Design review of the part built by this model. Coordinates are the model's own, in mm. Face numbers are marked on the shaded views. A direction names the side the tool comes from. Coordinates: 2 decimals unless noted, no trailing zeros. Order: outer loops, then holes, each group sorted by start corner. A loop starts at its lowest first (then second) coordinate and runs counter-clockwise, first axis right, second up. Notation, with made-up numbers: (-33, 39.25) - (19, 39.25) arc R8 ccw to (19, 48.25) - close; hole circle Ø4 at (46, 44). An arc over 180 degrees is marked (long way). Write each question's results on one line, items separated by ' | '. Start each with the question number.
```python
from build123d import *

# Parameters (mm, degrees)
SKETCH3_W           = 42.3
SKETCH3_H           = 42.3
BOSS_EXTRUDE1_DEPTH = 20.95
SKETCH4_R           = 4.05
CUT_EXTRUDE1_DEPTH  = 5
SKETCH5_R           = 2.5
CUT_EXTRUDE2_DEPTH  = 8.5
SKETCH6_R           = 3.05
BOSS_EXTRUDE2_DEPTH = 5
SKETCH7_R           = 2.05
CUT_EXTRUDE3_DEPTH  = 20
CHAMFER1_SIZE       = 4
CHAMFER3_SIZE       = 1
CUT_EXTRUDE4_DEPTH  = 1


with BuildPart() as part:
    # Sketch3 → Boss-Extrude1 (new body)
    with BuildSketch(Plane.XY):
        Rectangle(SKETCH3_W, SKETCH3_H)
    extrude(amount=BOSS_EXTRUDE1_DEPTH)

    # Sketch4 → Cut-Extrude1 (cut)
    with BuildSketch(Plane.XZ.offset(21.15)):
        with Locations(Location((0, 12.45, 0), (0, 0, 270))):
            Circle(SKETCH4_R)
    extrude(amount=-CUT_EXTRUDE1_DEPTH, mode=Mode.SUBTRACT)

    # Sketch5 → Cut-Extrude2 (cut)
    with BuildSketch(Plane.XY):
        Circle(SKETCH5_R)
    extrude(amount=CUT_EXTRUDE2_DEPTH, mode=Mode.SUBTRACT)

    # Sketch6 → Boss-Extrude2 (add)
    with BuildSketch(Plane(origin=(0, 21.15, 0), x_dir=(1, 0, 0), z_dir=(0, 1, 0))):
        with Locations(Location((0, -12.45, 0), (0, 0, 90))):
            Circle(SKETCH6_R)
    extrude(amount=BOSS_EXTRUDE2_DEPTH)

    # Sketch7 → Cut-Extrude3 (cut)
    with BuildSketch(Plane(origin=(0, 26.15, 0), x_dir=(1, 0, 0), z_dir=(0, 1, 0))):
        with Locations(Location((0, -12.45, 0), (0, 0, 270))):
            Circle(SKETCH7_R)
    extrude(amount=-CUT_EXTRUDE3_DEPTH, mode=Mode.SUBTRACT)

    # Chamfer1
    chamfer1_edges = [part.edges().sort_by_distance(p)[0] for p in [
        (21.15, 21.15, 10.475),
        (-21.15, 21.15, 10.475),
    ]]
    chamfer(chamfer1_edges, length=CHAMFER1_SIZE)

    # Chamfer3
    chamfer3_edges = [part.edges().sort_by_distance(p)[0] for p in [
        (0, 21.15, 15.5),
        (0, 26.15, 10.4),
    ]]
    chamfer(chamfer3_edges, length=CHAMFER3_SIZE - 0.0001)  # a hair under: the kernel refuses the full size

    # Sketch10 → Cut-Extrude4 (cut)
    with BuildSketch(Plane.XY.offset(20.95)):
        Polygon((19.15, -19.15), (19.15, 16.321572875), (16.321572875, 19.15), (-16.321572875, 19.15), (-19.15, 16.321572875), (-19.15, -19.15), align=None)
    extrude(amount=-CUT_EXTRUDE4_DEPTH, mode=Mode.SUBTRACT)


solid = part.part
```
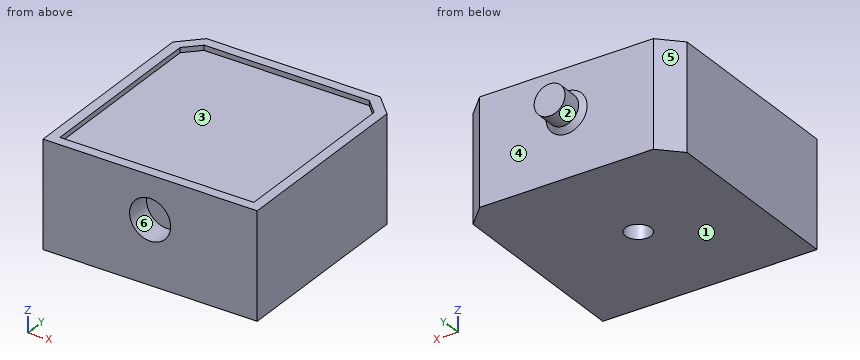
(1) Tool access review of the marked faces 1 and 2: name each direction out of +Z, -Z, +X, -X, +Y, -Y from which nothing blocks a thin tool from reaching the whole face with its end or side.
(2) Clearance check with flat-ended pins moving along their axes: pin 1 (1.5 mm diameter, centred on x = 14.5, y = -9.5, fed in from +Z); pin 2 (1.5 mm diameter, centred on x = -1, y = -0.5, fed in from -Z); pin 3 (1 mm diameter, centred on x = 15.5, y = -13.5, fed in from -Z); pin 4 (1.1 mm diameter, centred on x = 0, z = 20.5, fed in from +Y). State where each tip first meets the part, or that it passes through.
(3) Take a section at C-C (z = 2.25). State the section outline as (x, y) points.
(4) To check wall thickness, follow line 1 along X through (y, z) = (-19.8, 12.45); line 2 along Z through (x, y) = (12, 4); line 3 along Y through (x, z) = (0, 4.5). State the ranges of each line that lie inside material, in increasing order. Write a range as [from, to].
(5) Mouldability with a two-part tool opening along X and no side actions: class the marked faces 3, 4, 5 and 6 as +X half, -X half, draft (parallel to the pull), parting line (faces both ways), or undercut.
(6) Take a section at A-A (y = -12). State the section outline as (x, z) points.
(7) Take a section at D-D (y = 15). State the section outline as (x, z) points.
Worked out:
1) face 1: -Z, +X, -X, +Y, -Y | face 2: +Y
2) pin 1: z = 19.95 | pin 2: z = 8.5 | pin 3: z = 0 | pin 4: y = 21.15
3) outline: (-21.15, -21.15) - (21.15, -21.15) - (21.15, 17.15) - (17.15, 21.15) - (-17.15, 21.15) - (-21.15, 17.15) - close; hole circle Ø5 at (0, 0)
4) line 1: [-21.15, -4.05], [4.05, 21.15] | line 2: [0, 19.95] | line 3: [-21.15, -2.5], [2.5, 21.15]
5) face 3: undercut | face 4: draft | face 5: -X half | face 6: undercut
6) outline: (-21.15, 0) - (21.15, 0) - (21.15, 20.95) - (19.15, 20.95) - (19.15, 19.95) - (-19.15, 19.95) - (-19.15, 20.95) - (-21.15, 20.95) - close
7) outline: (-21.15, 0) - (21.15, 0) - (21.15, 20.95) - (19.15, 20.95) - (19.15, 19.95) - (-19.15, 19.95) - (-19.15, 20.95) - (-21.15, 20.95) - close; hole circle Ø4.1 at (0, 12.45)
